Input: part model. Units: mm. Frame: model coordinates. Round coordinates to 2 decimals unless told otherwise and drop trailing zeros. Loops run counter-clockwise (first coordinate to the right, second up) from the corner with the lowest first, then second, coordinate; pieces in that order, holes last. Notation, with made-up numbers: (-9.5, 28.5) -> (16.5, 28.5) arc R26 cw to (16.5, 59.5) -> close; hole circle Ø11 at (-26.75, 34). An arc over 180 degrees is marked (long way). Answer in a Markdown table with one row per item. Add a question column.
Q1. Section A-A, the plane y = 0. Output: boundary loops of the cut face in (x, z).
Q2. Ray query, L1, parallel to Z at x = 621, y = 0.5; L2, parallel to Y at x = 674, z = -1; L3, parallel to X at y = 7, z = 1.75. Return the intervals inside material, ascending. Write a range as from..to.
Q3. Pin query (flat end, axial travel): pin 1 (2 mm diameter, centred on x = 180.5, z = 5, fed in from -Y); pin 2 (1 mm diameter, centred on x = 619.5, z = -5, fed in from -Y); pin 3 (1.5 mm diameter, centred on x = 192, z = 3.5, fed in from -Y). Return the tip coordinate at first contact, or that it passes through.
Q4. Section C-C, the plane x = 769. Output: boundary loops of the cut face in (y, z).
Autodesk Inventor part; units mm, degrees
ref_plane "YZ Plane" through (0, 0, 0) normal (1, 0, 0) x (0, 1, 0)
ref_plane "XZ Plane" through (0, 0, 0) normal (0, 1, 0) x (-1, 0, 0)
ref_plane "XY Plane" through (0, 0, 0) normal (0, 0, 1) x (1, 0, 0)
sketch "Sketch1" plane through (0, 0, 0) normal (0, 0, 1) x (1, 0, 0)
  line L0 (0, 0) -> (0, 5)
  line L1 (0, 5) -> (15, 5)
  line L2 (15, 5) -> (15, 6)
  line L3 (15, 6) -> (54, 6)
  line L4 (54, 6) -> (54, 8)
  line L5 (54, 8) -> (1089, 8)
  line L6 (1089, 8) -> (1089, 5)
  line L7 (1089, 5) -> (1100, 5)
  line L8 (1100, 5) -> (1100, 0)
  line L9 (1100, 0) -> (0, 0)
  line L10 (0, 0) -> (1100, 0)
  dimension "d0" = 5
  dimension "d1" = 6
  dimension "d2" = 8
  dimension "d3" = 5
  dimension "d4" = 11
  dimension "d6" = 39
  dimension "d8" = 15
  dimension "d9" = 1100
revolve "Revolution1" add sketch "Sketch1" angle 360 about axis through (0, 0, 0) along (1, 0, 0)
properties part number "SFU1605"
Answer block:
| question | item | result |
|---|---|---|
| 1 | outline | (0, -5) -> (15, -5) -> (15, -6) -> (54, -6) -> (54, -8) -> (1089, -8) -> (1089, -5) -> (1100, -5) -> (1100, 5) -> (1089, 5) -> (1089, 8) -> (54, 8) -> (54, 6) -> (15, 6) -> (15, 5) -> (0, 5) -> close |
| 2 | L1 | -7.98..7.98 |
| 2 | L2 | -7.94..7.94 |
| 2 | L3 | 54..1089 |
| 3 | pin 1 | y = -6.93 |
| 3 | pin 2 | y = -6.61 |
| 3 | pin 3 | y = -7.51 |
| 4 | outline | circle Ø16 at (0, 0) |
